```python
from build123d import *

# Parameters (mm, degrees)
PAD_DEPTH = 10
FILLET_R  = 1


with BuildPart() as part:
    # Sketch → Pad (new body)
    with BuildSketch(Plane.XY):
        with BuildLine():
            ThreePointArc((24.115555, 15), (0, 28.4), (-24.115555, 15))
            ThreePointArc((-4.582576, 18.4), (-14.877009, 19.733033), (-24.115555, 15))
            ThreePointArc((4.582576, 18.4), (0, 25.4), (-4.582576, 18.4))
            ThreePointArc((24.115555, 15), (14.877009, 19.733033), (4.582576, 18.4))
        make_face()
    extrude(amount=PAD_DEPTH)

    # Fillet
    fillet_edges = [part.edges().sort_by_distance(p)[0] for p in [
        (-24.115555, 15, 5),
        (-4.582576, 18.4, 5),
        (4.582576, 18.4, 5),
        (24.115555, 15, 5),
    ]]
    fillet(fillet_edges, radius=FILLET_R)


solid = part.part
```
The listing builds one solid part. Answer for the finished solid, in the listing's coordinates (mm). Coordinates: 2 decimals unless noted, no trailing zeros. Loops run counter-clockwise (first coordinate to the right, second up) from the corner with the lowest first, then second, coordinate; pieces in that order, holes last. Notation, with made-up numbers: (60, 45.25) -> (72, 45.25) arc R33 ccw to (72, 81.25) -> close; hole circle Ø8 at (6, -15.5). An arc over 180 degrees is marked (long way). Return JSON: item names as keys, results as strings. Group by question number.
(1) Find the intervals of material crossed by probe 1 along X at (y, z) = (24, 5.75); probe 2 along X at (y, z) = (21, 1); probe 3 along X at (y, z) = (26.25, 3), in increasing order. Write a range as from..to.
(2) A cutting plane is placed at C-C on y = 27.5. Write down the section's boundary in (x, z).
(3) Given pin 1 Ø3 at (y, z) = (21, 1.5) entering from -X; pin 2 Ø1.5 at (x, z) = (11.5, 7) entering from -Y; pin 3 Ø1.5 at (x, z) = (5.5, 1) entering from -Y, each flat-ended and moving along its own axis, determine where each tip first touches the part or whether it passes through.
(4) Determine the mould class of faces 1 (the cylindrical face through (0.1, 25.4, 4.9)), 2 (the cylindrical face through (0.3, 28.4, 4.9)), 3 (the flat face through (0, 26, 0)) for opening direction X: released by +X, released by -X, zero draft, split by the parting line, or undercut.
(5) A cutting plane is placed at A-A on y = 23.5. Write down the section's boundary in (x, z), and give its area (3 significant figures).
(6) A cutting plane is placed at B-B on x = 0. Write down the section's boundary in (y, z), and give its area (3 significant figures).
The answers:
{
 "1": {"probe 1": "x = -15.18..-3.47, 3.47..15.18", "probe 2": "x = -19.12..-4.96, 4.96..19.12", "probe 3": "x = -10.84..10.84"},
 "2": {"outline": "(-7.09, 0) -> (7.09, 0) -> (7.09, 10) -> (-7.09, 10) -> close"},
 "3": {"pin 1": "stops at x = -20.32", "pin 2": "stops at y = 19.96", "pin 3": "stops at y = 19.03"},
 "4": {"face 1": "undercut", "face 2": "split by the parting line", "face 3": "zero draft"},
 "5": {"outline": "(-15.95, 0) -> (-3.92, 0) -> (-3.92, 10) -> (-15.95, 10) -> close; (3.92, 0) -> (15.95, 0) -> (15.95, 10) -> (3.92, 10) -> close", "area": "240 mm^2"},
 "6": {"outline": "(25.4, 0) -> (28.4, 0) -> (28.4, 10) -> (25.4, 10) -> close", "area": "30.0 mm^2"}
}
